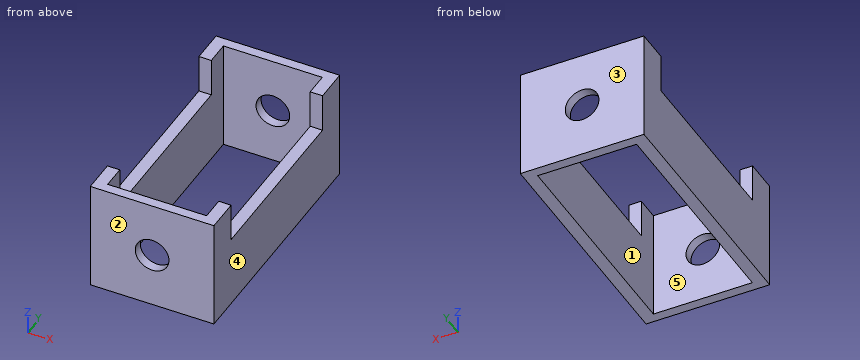
from build123d import *

# Parameters (mm, degrees)
F0_W     = 56.617882
F0_H     = 111.745812
F0_W_2   = 45.294308
F0_H_2   = 102.806144
F1_DEPTH = 50.8
F3_DEPTH = 76.2
F4_R     = 7.715563
F5_DEPTH = 127


with BuildPart() as f1:
    # F0 (on Top) → F1 (new body)
    with BuildSketch(Plane.XY):
        Rectangle(F0_W, F0_H)
        Rectangle(F0_W_2, F0_H_2, mode=Mode.SUBTRACT)
    extrude(amount=F1_DEPTH)

    # F2 (on face) → F3 (cut)
    with BuildSketch(Plane.YZ.offset(28.308941)):
        Polygon((40.64, 50.8), (0, 50.8), (-40.64, 50.8), (-40.64, 33.02), (40.64, 33.02), align=None)
    extrude(amount=-F3_DEPTH, mode=Mode.SUBTRACT)

    # F4 (on face) → F5 (cut)
    with BuildSketch(Plane.XZ.offset(55.872906)):
        with Locations((0, 25.4)):
            Circle(F4_R)
    extrude(amount=-F5_DEPTH, mode=Mode.SUBTRACT)


solid = f1.part
Here's how the part is built. I have some questions about the finished solid (model axes, mm). Face numbers are marked on the shaded views. A direction names the side the tool comes from. Coordinates: 2 decimals unless noted, no trailing zeros. Order: outer loops, then holes, each group sorted by start corner. A loop starts at its lowest first (then second) coordinate and runs counter-clockwise, first axis right, second up. Notation, with made-up numbers: (80.5, 72) - (85.5, 72) arc R33 cw to (85.5, 109) - close; hole circle Ø10 at (13, 7). An arc over 180 degrees is marked (long way). Use CSV: the item, a comma, the result in double quotes. Start each with the question number.
1. Suppose I cut it at D-D on x = 18.5. List the corners of the cut face in (y, z) for me, then the cut area to 3 significant figures.
2. Suppose I cut it at B-B on z = 37. List the corners of the cut face in (x, y) for me, then the cut area to 3 significant figures.
3. I'm going to push a flat-ended pin straight in: pin 1 (1.7 mm diameter, centred on x = 25.5, y = -16.5, fed in from +Z). Where does the tip first touch, or does it pass through?
4. If we mould it in two halves opening along Y, with no side actions, what happens to the marked faces 3, 4 and 5? For each: +Y half, -Y half, draft (parallel to the pull), parting line (faces both ways), or undercut.
5. Please list where these lines run through material, in increasing order: line 1 (X direction, y = -2.5, z = 31); line 2 (Y direction, x = -20, z = 42); line 3 (Z direction, x = 0, y = 54.8). Write a range as from..to.
6. For the marked faces 1 and 2, which set-ups out of +Z, -Z, +X, -X, +Y, -Y let a thin tool reach every point of the face, with its end or its side?
7. Suppose I cut it at A-A on x = 0. List the corners of the cut face in (y, z) for me, then the cut area to 3 significant figures.
8. Suppose I cut it at C-C on y = 42. List the corners of the cut face in (x, z) for me, then the cut area to 3 significant figures.
Output:
1,outline,"(-55.87, 0) - (-51.4, 0) - (-51.4, 50.8) - (-55.87, 50.8) - close; (51.4, 0) - (55.87, 0) - (55.87, 50.8) - (51.4, 50.8) - close"
1,area,"454 mm2"
2,outline,"(-28.31, -55.87) - (28.31, -55.87) - (28.31, -40.64) - (22.65, -40.64) - (22.65, -51.4) - (-22.65, -51.4) - (-22.65, -40.64) - (-28.31, -40.64) - close; (-28.31, 40.64) - (-22.65, 40.64) - (-22.65, 51.4) - (22.65, 51.4) - (22.65, 40.64) - (28.31, 40.64) - (28.31, 55.87) - (-28.31, 55.87) - close"
2,area,"750 mm2"
3,pin 1,"stops at z = 33.02"
4,face 3,"+Y half"
4,face 4,"draft"
4,face 5,"undercut"
5,line 1,"x = -28.31..-22.65, 22.65..28.31"
5,line 2,"y = -55.87..-51.4, 51.4..55.87"
5,line 3,"z = 0..17.68, 33.12..50.8"
6,face 1,"+Z, -Z"
6,face 2,"+Z, -Z, +X, -X, -Y"
7,outline,"(-55.87, 0) - (-51.4, 0) - (-51.4, 17.68) - (-55.87, 17.68) - close; (-55.87, 33.12) - (-51.4, 33.12) - (-51.4, 50.8) - (-55.87, 50.8) - close; (51.4, 0) - (55.87, 0) - (55.87, 17.68) - (51.4, 17.68) - close; (51.4, 33.12) - (55.87, 33.12) - (55.87, 50.8) - (51.4, 50.8) - close"
7,area,"316 mm2"
8,outline,"(-28.31, 0) - (-22.65, 0) - (-22.65, 50.8) - (-28.31, 50.8) - close; (22.65, 0) - (28.31, 0) - (28.31, 50.8) - (22.65, 50.8) - close"
8,area,"575 mm2"
